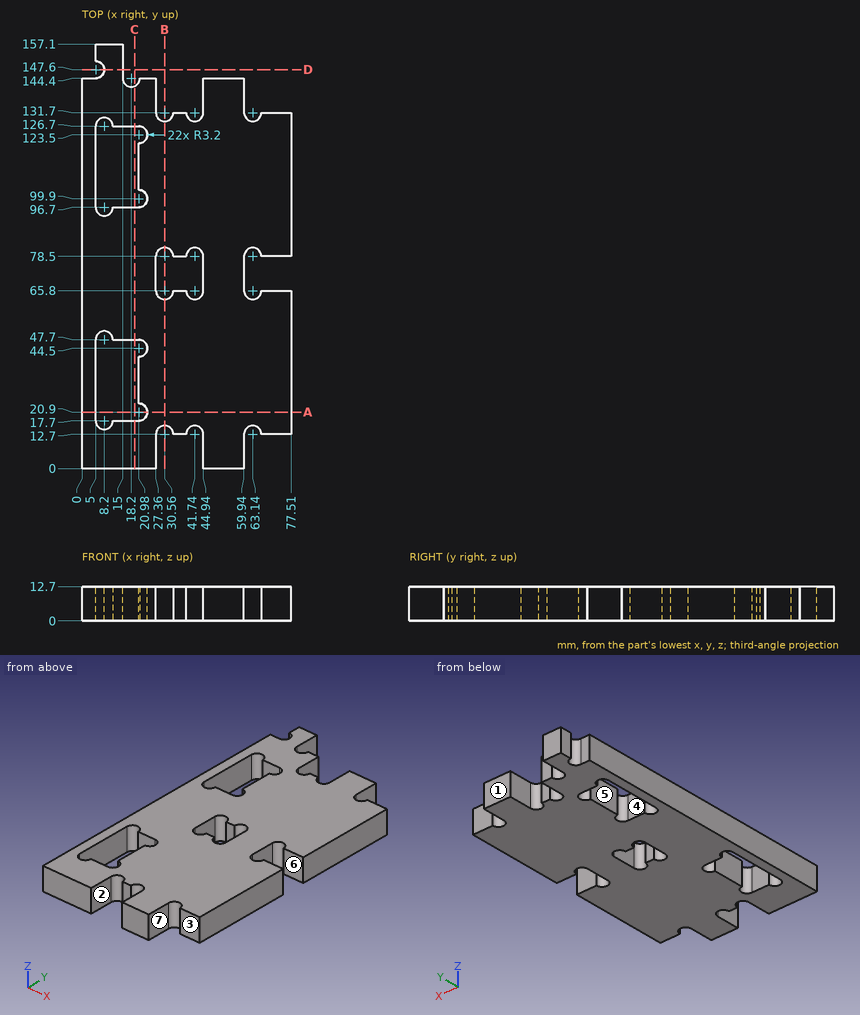
Can you work these out from the drawing? Everything is in mm from the part's minimum corner. A direction names the side the tool comes from. Give positions to 0.01 mm unless a question says otherwise; leave off trailing zeros. Loops run counter-clockwise (first coordinate to the right, second up) from the corner with the lowest first, then second, coordinate; pieces in that order, holes last. Notation, with made-up numbers: (9, 8) -> (18, 8) arc R13 ccw to (18, 14) -> close; hole circle Ø7 at (85, 72.5). An arc over 180 degrees is marked (long way). Return JSON: item names as keys, results as strings.
Item 1: I need wall thicknesses on L1, parallel to Y at x = 12, z = 1.5; L2, parallel to X at y = 65.5, z = 3.5; L3, parallel to Y at x = 70.5, z = 7.75. Which ranges of each line are inside material? Lowest first, please. Write a range as from..to.
Geometry results:
{"L1": "y = 0..17.7, 47.7..96.7, 126.7..157.1", "L2": "x = 0..27.37, 33.75..38.55, 44.93..59.95, 66.33..77.51", "L3": "y = 12.7..65.8, 78.5..131.7"}
Item 2: Which directions (+Z, -Z, +X, -X, +Y, -Y) give clear straight access to the entire face, cutting with the end or side of a thin tool? Please do the marked faces 1, 2, 3 and 4.
Geometry results:
{"face 1": "+Z, -Z, +X, +Y", "face 2": "+Z, -Z, -Y", "face 3": "+Z, -Z, +X, -Y", "face 4": "+Z, -Z"}
Item 3: If we section it at C-C on x = 19.5: List the corners of the cut face in (y, z) for me, plus the area to 3 significant figures.
Geometry results:
{"outline": "(0, 0) -> (17.7, 0) -> (17.7, 12.7) -> (0, 12.7) -> close; (47.7, 0) -> (96.7, 0) -> (96.7, 12.7) -> (47.7, 12.7) -> close; (126.7, 0) -> (141.48, 0) -> (141.48, 12.7) -> (126.7, 12.7) -> close", "area": "1,030 mm²"}
Item 4: If we section it at D-D on y = 147.6: List the corners of the cut face in (x, z) for me.
Geometry results:
{"outline": "(8.2, 0) -> (15, 0) -> (15, 12.7) -> (8.2, 12.7) -> close"}
Item 5: I'm going to push flat-ended pins straight in: pin 1 (4 mm diameter, centred on y = 138, z = 5.5, fed in from +X); pin 2 (1.4 mm diameter, centred on x = 36, z = 6, fed in from +Y); pin 3 (5.5 mm diameter, centred on x = 71.5, z = 3.5, fed in from -Y). Where does each tip first touch, or does it pass through?
Geometry results:
{"pin 1": "stops at x = 59.94", "pin 2": "stops at y = 131.7", "pin 3": "stops at y = 12.7"}
Item 6: If we section it at B-B on x = 30.56: List the corners of the cut face in (y, z) for me.
Geometry results:
{"outline": "(15.9, 0) -> (62.6, 0) -> (62.6, 12.7) -> (15.9, 12.7) -> close; (81.7, 0) -> (128.5, 0) -> (128.5, 12.7) -> (81.7, 12.7) -> close"}
Item 7: If we section it at A-A on y = 20.9: List the corners of the cut face in (x, z) for me, plus the area to 3 significant figures.
Geometry results:
{"outline": "(0, 0) -> (5, 0) -> (5, 12.7) -> (0, 12.7) -> close; (24.18, 0) -> (77.51, 0) -> (77.51, 12.7) -> (24.18, 12.7) -> close", "area": "741 mm²"}
Item 8: We'd pull the mould along X, two halves only. Please class the marked faces 5, 6 and 7: +X half, -X half, draft (parallel to the pull), parting line (faces both ways), or undercut.
Geometry results:
{"face 5": "undercut", "face 6": "draft", "face 7": "+X half"}
